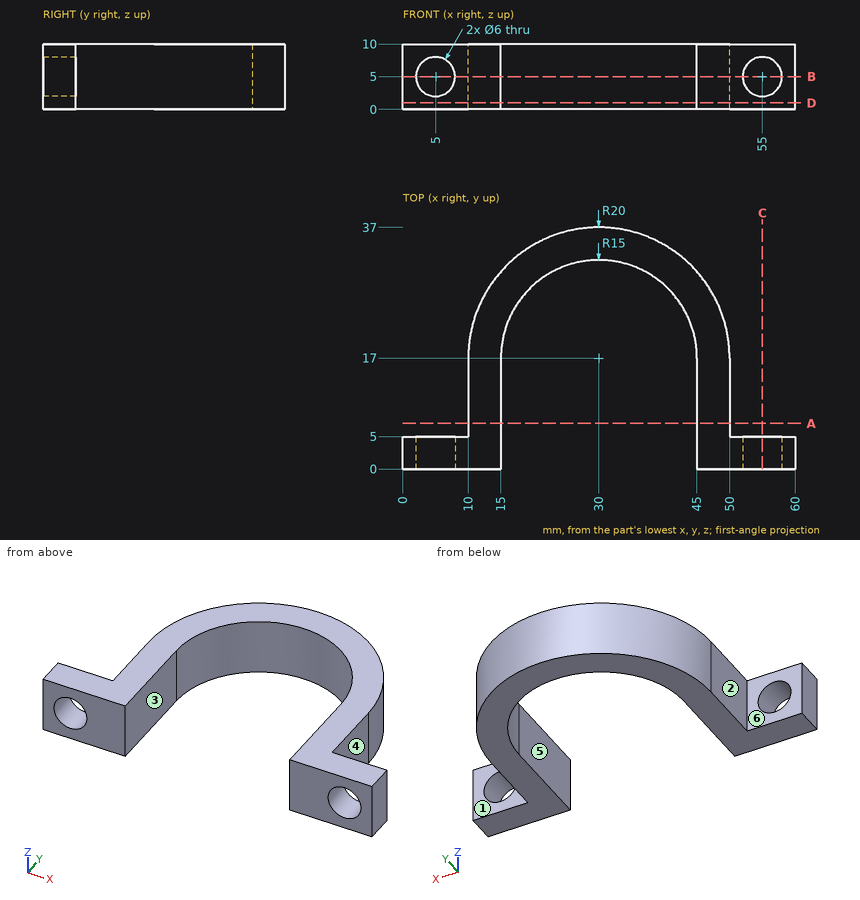
Part print with two shaded views. Sizes in mm from the minimum x, y, z corner. A direction names the side the tool comes from. Coordinates: 2 decimals unless noted, no trailing zeros. Order: outer loops, then holes, each group sorted by start corner. A loop starts at its lowest first (then second) coordinate and runs counter-clockwise, first axis right, second up. Notation, with made-up numbers: (-30, 32.5) - (-14, 32.5) arc R30 cw to (-14, 63.5) - close; hole circle Ø1 at (55, 75). An arc over 180 degrees is marked (long way). Write item = value, one per line. Start each with the question number.
1) Saw through at D-D on z = 1. Write the cut outline in (x, y).
2) Saw through at B-B on z = 5. Write the cut outline in (x, y), then the cut area to 3 significant figures.
3) Two-plate mould, pull along X, no slides. Class the marked faces 4, 5 and 6: pulls with the +X half, pulls with the -X half, needs draft (parallel to the pull), parting line crosses it, or undercut.
4) Wall check: line 1 along X through (y, z) = (2.8, 5); line 2 along X through (y, z) = (13, 9.75); line 3 along Z through (x, y) = (5, 2.7). Give the ranges that are in metal, low to high. Write a range as from..to.
5) 3-axis set-ups, long thin cutter, end or side, ignore diameter. For the marked faces 1, 2 and 3: which of +Z, -Z, +X, -X, +Y, -Y reach the whole face in a straight line?
6) Saw through at C-C on x = 55. Write the cut outline in (y, z), then the cut area to 3 significant figures.
7) Flat gauge pins, fed straight in: pin 1 Ø1.5 at (y, z) = (22.5, 7) entering from +X; pin 2 Ø5 at (y, z) = (24, 4.5) entering from -X; pin 3 Ø5 at (y, z) = (19.5, 6.5) entering from +X; pin 4 Ø5 at (x, y) = (11.5, 24.5) entering from -Z. Where does each tip first touch, or does it go through?
8) Saw through at A-A on y = 7. Write the cut outline in (x, z), then the cut area to 3 significant figures.
From the geometry:
q1.outline = (0, 0) - (15, 0) - (15, 17) arc R15 cw to (45, 17) - (45, 0) - (60, 0) - (60, 5) - (50, 5) - (50, 17) arc R20 ccw to (10, 17) - (10, 5) - (0, 5) - close
q2.outline = (0, 0) - (2, 0) - (2, 5) - (0, 5) - close; (8, 0) - (15, 0) - (15, 17) arc R15 cw to (45, 17) - (45, 0) - (52, 0) - (52, 5) - (50, 5) - (50, 17) arc R20 ccw to (10, 17) - (10, 5) - (8, 5) - close; (58, 0) - (60, 0) - (60, 5) - (58, 5) - close
q2.area = 485 mm^2
q3.face_4 = pulls with the +X half
q3.face_5 = undercut
q3.face_6 = needs draft
q4.line_1 = 0..2, 8..15, 45..52, 58..60
q4.line_2 = 10..15, 45..50
q4.line_3 = 0..2, 8..10
q5.face_1 = +Z, -Z, +X, +Y
q5.face_2 = +Z, -Z, -X, +Y
q5.face_3 = +Z, -Z, -Y
q6.outline = (0, 0) - (5, 0) - (5, 2) - (0, 2) - close; (0, 8) - (5, 8) - (5, 10) - (0, 10) - close
q6.area = 20.0 mm^2
q7.pin_1 = 49.43
q7.pin_2 = 10.51
q7.pin_3 = 50
q7.pin_4 = 0
q8.outline = (10, 0) - (15, 0) - (15, 10) - (10, 10) - close; (45, 0) - (50, 0) - (50, 10) - (45, 10) - close
q8.area = 100 mm^2
